The model under review builds one solid part; all positions refer to its coordinate system, in mm. Face numbers are marked on the shaded views. A direction names the side the tool comes from. Coordinates: 2 decimals unless noted, no trailing zeros. Write each loop counter-clockwise with the first axis right and the second up, starting at its lowest first coordinate (ties: lowest second). Pieces come first, ordered by that corner, then holes. Notation, with made-up numbers: (35.5, 3.25) - (77.5, 3.25) arc R26 ccw to (77.5, 38.25) - close; hole circle Ø11 at (32.25, 57.25). An arc over 180 degrees is marked (long way). Put each result on its own line as item: value.
from build123d import *

# Parameters (mm, degrees)
SKETCH1_R          = 3.9
EXTRUDE1_DEPTH     = 22.4
SKETCH2_R          = 3
EXTRUDE2_DEPTH     = 12.5
SKETCH3_R          = 5.5
EXTRUDE3_DEPTH     = 2.4
CHAMFER1_SIZE      = 0.75
SKETCH4_W          = 11
SKETCH4_H          = 1.6
CUT_EXTRUDE1_DEPTH = 1.75
CHAMFER2_SIZE      = 0.75


with BuildPart() as part:
    # Sketch1 → Extrude1 (new body)
    with BuildSketch(Plane.XY):
        Circle(SKETCH1_R)
    extrude(amount=-EXTRUDE1_DEPTH)

    # Sketch2 → Extrude2 (add)
    with BuildSketch(Plane(origin=(0, 0, -22.4), x_dir=(-1, 0, 0), z_dir=(0, 0, -1))):
        with Locations(Location((0, 0, 0), (0, 0, 180))):
            Circle(SKETCH2_R)
    extrude(amount=EXTRUDE2_DEPTH)

    # Sketch3 → Extrude3 (add)
    with BuildSketch(Plane.XY):
        Circle(SKETCH3_R)
    extrude(amount=EXTRUDE3_DEPTH)

    # Chamfer1
    chamfer1_edges = [part.edges().sort_by_distance(p)[0] for p in [
        (-3, 0, -34.9),
    ]]
    chamfer(chamfer1_edges, length=CHAMFER1_SIZE)

    # Sketch4 → Cut-Extrude1 (cut)
    with BuildSketch(Plane.XY.offset(2.4)):
        Rectangle(SKETCH4_W, SKETCH4_H)
    extrude(amount=-CUT_EXTRUDE1_DEPTH, mode=Mode.SUBTRACT)

    # Chamfer2
    chamfer2_edges = [part.edges().sort_by_distance(p)[0] for p in [
        (0, 5.5, 2.4),
        (0, -5.5, 2.4),
    ]]
    chamfer(chamfer2_edges, length=CHAMFER2_SIZE)


solid = part.part
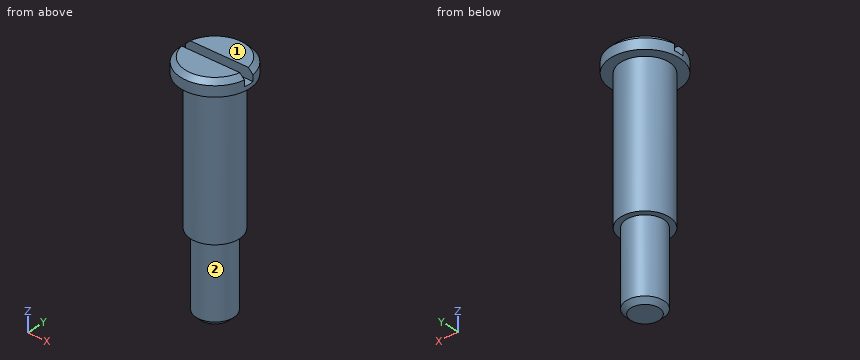
1. Machinability: for the marked faces 1 and 2, which of the approach directions +Z, -Z, +X, -X, +Y, -Y give a long, thin tool a straight path to every point of the face, cutting with its end or side? Answer none if there is none.
Determined:
face 1: +Z, +X, -X, +Y, -Y
face 2: -Z
2. For pin 1 Ø5 at (x, z) = (-4, -12.5) entering from +Y; pin 2 Ø0.9 at (x, z) = (-1, 1.5) entering from +Y; pin 3 Ø1.9 at (x, z) = (2.5, 1.5) entering from -Y, all flat-tipped, find the tip position at first contact; note any pin that passes through.
Determined:
pin 1: stops at y = 3.6
pin 2: stops at y = 5.47
pin 3: stops at y = -5.28
3. Consider section B-B on y = 0. State the section outline as (x, z) points, plus the area to 3 significant figures.
Determined:
outline: (-5.5, 0) - (-3.9, 0) - (-3.9, -22.4) - (-3, -22.4) - (-3, -34.15) - (-2.25, -34.9) - (2.25, -34.9) - (3, -34.15) - (3, -22.4) - (3.9, -22.4) - (3.9, 0) - (5.5, 0) - (5.5, 0.65) - (-5.5, 0.65) - close
area: 256 mm^2
4. Consider section D-D on z = -30.5. State the section outline as (x, y) points.
Determined:
outline: circle Ø6 at (0, 0)
5. Consider section A-A on x = 0. State the section outline as (y, z) points.
Determined:
outline: (-5.5, 0) - (-3.9, 0) - (-3.9, -22.4) - (-3, -22.4) - (-3, -34.15) - (-2.25, -34.9) - (2.25, -34.9) - (3, -34.15) - (3, -22.4) - (3.9, -22.4) - (3.9, 0) - (5.5, 0) - (5.5, 1.65) - (4.75, 2.4) - (0.8, 2.4) - (0.8, 0.65) - (-0.8, 0.65) - (-0.8, 2.4) - (-4.75, 2.4) - (-5.5, 1.65) - close
6. Consider section C-C on z = -9. State the section outline as (x, y) points.
Determined:
outline: circle Ø7.8 at (0, 0)
7. To check wall thickness, follow probe 1 along Z at (x, y) = (4.75, -0.75); probe 2 along X at (y, z) = (-2.5, -1); probe 3 along Z at (x, y) = (4, -2). State the ranges of each line that lie inside material, in increasing order.
Determined:
probe 1: z = 0 to 0.65
probe 2: x = -2.99 to 2.99
probe 3: z = 0 to 2.4
